For this review, use the dimensioned drawing (mm, ordinates from the lowest corner) and the shaded views. A direction names the side the tool comes from. Round coordinates to 2 decimals unless told otherwise and drop trailing zeros. Loops run counter-clockwise (first coordinate to the right, second up) from the corner with the lowest first, then second, coordinate; pieces in that order, holes last. Notation, with made-up numbers: M -34,49 L 7,49 A20 ccw 7,56 Z; hole C 78,-22.5 d4. An arc over 180 degrees is marked long. One line per item, written item: value. Start each with the question number.
Item 1: Mouldability with a two-part tool opening along Y and no side actions: class the marked faces 1, 2, 3 and 4 as released by +Y, released by -Y, zero draft, split by the parting line, or undercut.
Item 2: We need section B-B (y = 9.5). State how many separate pieces and enclosed holes the cut face has.
Item 3: For the marked faces 5 and 6, list the 3-axis set-ups (+Z, -Z, +X, -X, +Y, -Y) from which the entire face can be reached by the end or side of a thin tool; tool diameter is ignored.
Item 4: Clearance check with flat-ended pins moving along their axes: pin 1 (12 mm diameter, centred on x = 20, z = 21, fed in from -Y); pin 2 (2 mm diameter, centred on x = 14, z = 22, fed in from -Y) (3 decimals); pin 3 (1 mm diameter, centred on y = 13, z = 0.5, fed in from -X); pin 4 (6 mm diameter, centred on x = 7.5, z = 22, fed in from +Y). State where each tip first meets the part, or that it passes through.
Item 5: We need section C-C (x = 32). Write out the cut boundary in (y, z) (1 decimal).
Item 6: For line 1 along X through (y, z) = (5, 8.5) (1 decimal); line 2 along Z through (x, y) = (22.5, 9.5); line 3 along Y through (x, z) = (42, 3.75), list the stretches that pass through material, from the lowest coordinate up.
Item 7: We need section A-A (z = 3). Write out the cut boundary in (x, y), then the cut area to 3 significant figures.
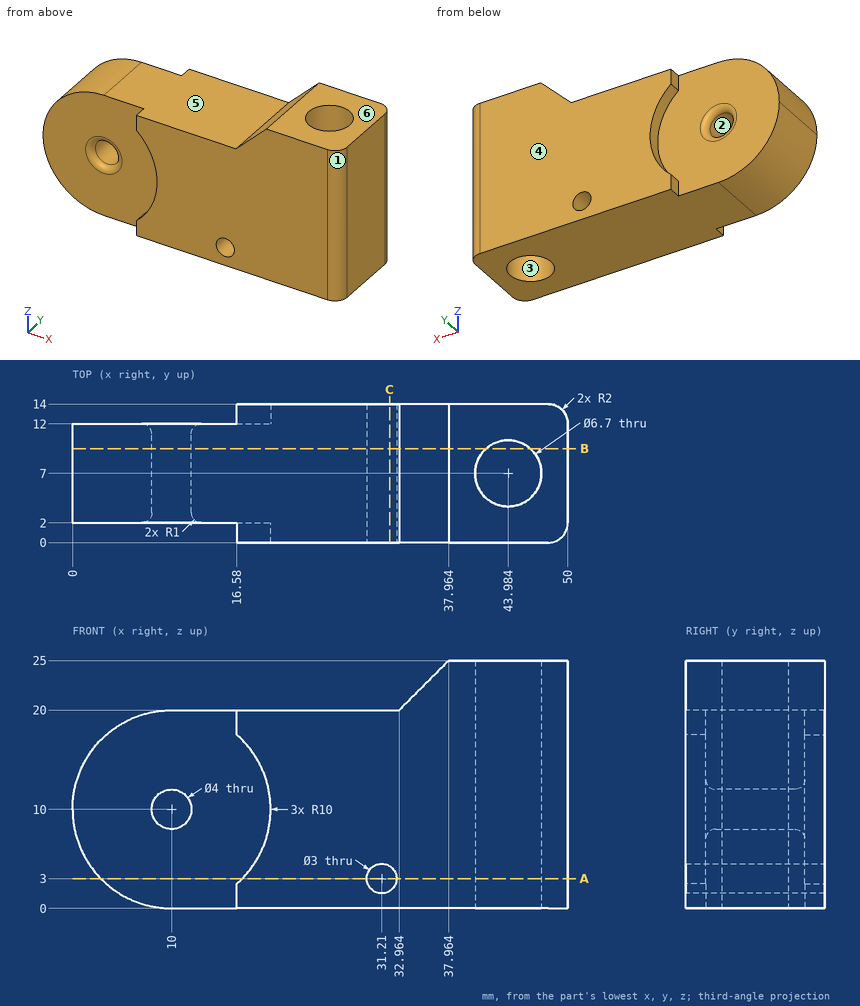
A:
1. face 1: released by -Y
1. face 2: zero draft
1. face 3: undercut
1. face 4: released by +Y
2. separate pieces: 2
2. enclosed holes: 2
3. face 5: +Z, -X, +Y, -Y
3. face 6: +Z, +X, -X, +Y, -Y
4. pin 1: y = 0
4. pin 2: through
4. pin 3: x = 16.58
4. pin 4: y = 12
5. outline: M 0,0 L 14,0 L 14,1.7 L 0,1.7 Z; M 0,4.3 L 14,4.3 L 14,20 L 0,20 Z
6. line 1: 0.1 to 8.7, 11.3 to 41.3, 46.7 to 50
6. line 2: 0 to 20
6. line 3: 0 to 4.3, 9.7 to 14
7. outline: M 2.86,2 L 17.14,2 L 17.14,0 L 29.71,0 L 29.71,14 L 17.14,14 L 17.14,12 L 2.86,12 Z; M 32.71,0 L 48,0 A2 ccw 50,2 L 50,12 A2 ccw 48,14 L 32.71,14 Z; hole C 43.98,7 d6.7
7. area: 524 mm2
